For this review, take the finished solid that the model builds, in its own axes (mm). Give positions to 0.01 mm unless a question says otherwise; leave off trailing zeros. Write each loop counter-clockwise with the first axis right and the second up, starting at its lowest first coordinate (ties: lowest second). Pieces come first, ordered by that corner, then holes. Notation, with made-up numbers: M 10.25,37 L 31.25,37 A20 cw 31.25,73 Z; hole C 85.25,21.25 d1. An arc over 180 degrees is marked long. Use one line per item in the form item = value. Start each with the question number.
Q1. Consider section C-C on y = -12. Write out the cut boundary in (x, z).
Q2. Consider section A-A on x = -30.85. Write out the cut boundary in (y, z), and give its area (3 significant figures).
Q3. Consider section D-D on z = 15.4. Write out the cut boundary in (x, y), and give its area (3 significant figures).
Q4. Consider section B-B on z = 12.55. Write out the cut boundary in (x, y).
Q5. Clearance check with a flat-ended pin moving along its axis: pin 1 Ø1 at (y, z) = (-21.5, 15) entering from +X. State where the tip first meets the part, or that it passes through.
Q6. For probe 1 along X at (y, z) = (-2.5, 12.85); probe 2 along Z at (x, y) = (-31.1, -3.5); probe 3 along X at (y, z) = (-7.25, 14.6), list the stretches that pass through material, from the lowest coordinate up. Write a range as [from, to].
```python
from build123d import *

# Parameters (mm, degrees)
F1_DEPTH = 6
F2_DEPTH = 3
F3_DEPTH = 25
F4_DEPTH = 25


with BuildPart() as f1:
    # F0 (on Front) → F1 (new body)
    with BuildSketch(Plane.XZ):
        with BuildLine():
            ThreePointArc((-30.070162, 46.37237), (-35.632137, 46.568408), (-41.166509, 47.155549))
            ThreePointArc((-41.166509, 47.155549), (-30.070162, -22.199768), (-18.973814, 47.155549))
            ThreePointArc((-18.973814, 47.155549), (-24.508186, 46.568408), (-30.070162, 46.37237))
        make_face()
        with BuildLine():
            ThreePointArc((-22.570162, 13.365558), (-35.373463, 8.062257), (-30.070162, 20.865558))
            ThreePointArc((-30.070162, 20.865558), (-24.766861, 18.668859), (-22.570162, 13.365558))
        make_face(mode=Mode.SUBTRACT)
    extrude(amount=F1_DEPTH)

    # F0 (on Front) → F2 (join)
    with BuildSketch(Plane.XZ):
        with BuildLine():
            ThreePointArc((-30.070162, 56.279502), (-36.966771, 53.357463), (-41.166509, 47.155549))
            ThreePointArc((-41.166509, 47.155549), (-35.632137, 46.568408), (-30.070162, 46.37237))
            Line((-30.070162, 46.37237), (-30.070162, 50.721558))
            ThreePointArc((-30.070162, 50.721558), (-32.070162, 52.721558), (-30.070162, 54.721558))
            Line((-30.070162, 54.721558), (-30.070162, 56.279502))
        make_face()
        with BuildLine():
            ThreePointArc((-30.070162, 46.37237), (-24.508186, 46.568408), (-18.973814, 47.155549))
            ThreePointArc((-18.973814, 47.155549), (-23.173552, 53.357463), (-30.070162, 56.279502))
            Line((-30.070162, 56.279502), (-30.070162, 54.721558))
            ThreePointArc((-30.070162, 54.721558), (-28.655948, 54.135772), (-28.070162, 52.721558))
            ThreePointArc((-28.070162, 52.721558), (-28.655948, 51.307344), (-30.070162, 50.721558))
            Line((-30.070162, 50.721558), (-30.070162, 46.37237))
        make_face()
    extrude(amount=F2_DEPTH)


with BuildPart() as f3:
    # F0 (on Front) → F3 (new body)
    with BuildSketch(Plane.XZ):
        with BuildLine():
            ThreePointArc((-27.570162, 13.365558), (-28.302395, 15.133325), (-30.070162, 15.865558))
            ThreePointArc((-30.070162, 15.865558), (-31.837929, 11.597791), (-27.570162, 13.365558))
        make_face()
        with BuildLine():
            ThreePointArc((-28.570162, 13.365558), (-31.130822, 12.304898), (-30.070162, 14.865558))
            ThreePointArc((-30.070162, 14.865558), (-29.009502, 14.426218), (-28.570162, 13.365558))
        make_face(mode=Mode.SUBTRACT)
    extrude(amount=F3_DEPTH)


with BuildPart() as f4:
    # F0 (on Front) → F4 (new body)
    with BuildSketch(Plane.XZ):
        with BuildLine():
            ThreePointArc((-22.570162, 13.365558), (-24.766861, 18.668859), (-30.070162, 20.865558))
            ThreePointArc((-30.070162, 20.865558), (-35.373463, 8.062257), (-22.570162, 13.365558))
        make_face()
        with BuildLine():
            ThreePointArc((-27.570162, 13.365558), (-31.837929, 11.597791), (-30.070162, 15.865558))
            ThreePointArc((-30.070162, 15.865558), (-28.302395, 15.133325), (-27.570162, 13.365558))
        make_face(mode=Mode.SUBTRACT)
    extrude(amount=-F4_DEPTH)


solid = f3.part
```
Working result:
q1.outline = C -30.07,13.37 d5; hole C -30.07,13.37 d3
q2.outline = M -25,10.99 L 0,10.99 L 0,12.08 L -25,12.08 Z; M -25,14.65 L 0,14.65 L 0,15.74 L -25,15.74 Z
q2.area = 54.7 mm²
q3.outline = M -31.52,-25 L -28.62,-25 L -28.62,0 L -31.52,0 Z
q3.area = 72.6 mm²
q4.outline = M -32.43,-25 L -31.33,-25 L -31.33,0 L -32.43,0 Z; M -28.81,-25 L -27.71,-25 L -27.71,0 L -28.81,0 Z
q5.pin_1 = -27.84
q6.probe_1 = [-32.52, -31.48], [-28.66, -27.62]
q6.probe_2 = [11.09, 12.27], [14.46, 15.64]
q6.probe_3 = [-32.24, -30.92], [-29.22, -27.9]
